The listing builds one solid part. Answer for the finished solid, in the listing's coordinates (mm). A direction names the side the tool comes from. Give positions to 0.01 mm unless a question says otherwise; leave off trailing zeros. Order: outer loops, then holes, each group sorted by start corner. A loop starts at its lowest first (then second) coordinate and runs counter-clockwise, first axis right, second up.
```python
from build123d import *

# Parameters (mm, degrees)
SKETCH1_W           = 57
SKETCH1_H           = 5
BOSS_EXTRUDE1_DEPTH = 30
SKETCH2_W           = 30
SKETCH2_H           = 8
BOSS_EXTRUDE2_DEPTH = 47
SKETCH3_R           = 5
CUT_EXTRUDE1_DEPTH  = 80.737067917
SKETCH5_R           = 1.6
CUT_EXTRUDE3_DEPTH  = 14
FILLET1_R           = 5
FILLET2_R           = 5


with BuildPart() as part:
    # Sketch1 → Boss-Extrude1 (new body)
    with BuildSketch(Plane(origin=(0, 0, 0), x_dir=(0, 0, -1), z_dir=(1, 0, 0))):
        with Locations((28.5, 2.5)):
            Rectangle(SKETCH1_W, SKETCH1_H)
    boss_extrude1 = extrude(amount=BOSS_EXTRUDE1_DEPTH)

    # Sketch2 → Boss-Extrude2 (add)
    with BuildSketch(Plane(origin=(0, 5, 0), x_dir=(1, 0, 0), z_dir=(0, 1, 0))):
        with Locations((15, 53)):
            Rectangle(SKETCH2_W, SKETCH2_H)
    extrude(amount=BOSS_EXTRUDE2_DEPTH)

    # Sketch3 → Cut-Extrude1 (cut, through all)
    with BuildSketch(Plane(origin=(0, 5, 0), x_dir=(1, 0, 0), z_dir=(0, 1, 0))):
        with Locations(Location((15, 22, 0), (0, 0, 270))):
            Circle(SKETCH3_R)
    cut_extrude1 = extrude(amount=-CUT_EXTRUDE1_DEPTH, mode=Mode.SUBTRACT)

    # Sketch5 → Cut-Extrude3 (cut)
    with BuildSketch(Plane(origin=(0, 52, 0), x_dir=(1, 0, 0), z_dir=(0, 1, 0))):
        with Locations(Location((5, 53, 0), (0, 0, 270))):
            Circle(SKETCH5_R)
        with Locations(Location((25, 53, 0), (0, 0, 270))):
            Circle(SKETCH5_R)
    extrude(amount=-CUT_EXTRUDE3_DEPTH, mode=Mode.SUBTRACT)

    # Fillet1
    fillet1_edges = [part.edges().sort_by_distance(p)[0] for p in [
        (15, 5, -49),
        (30, 2.5, 0),
        (0, 2.5, 0),
        (15, 0, -57),
    ]]
    fillet(fillet1_edges, radius=FILLET1_R)

    # Mirror1: Boss-Extrude1, Cut-Extrude1 across plane
    add(boss_extrude1.mirror(Plane(origin=(0, 0, -53), x_dir=(1, 0, 0), z_dir=(0, 0, -1))))
    add(cut_extrude1.mirror(Plane(origin=(0, 0, -53), x_dir=(1, 0, 0), z_dir=(0, 0, -1))), mode=Mode.SUBTRACT)

    # Fillet2
    fillet2_edges = [part.edges().sort_by_distance(p)[0] for p in [
        (15, 5, -57),
        (0, 2.5, -106),
        (30, 2.5, -106),
    ]]
    fillet(fillet2_edges, radius=FILLET2_R)


solid = part.part
```
1) Straight lines are drawn through the part: probe 1 along X at (y, z) = (49, -53); probe 2 along X at (y, z) = (2, -22); probe 3 along Z at (x, y) = (20, 44.5). For each, find the intervals that lie inside material, in ascending order.
Geometry says:
probe 1: x = 0 to 3.4, 6.6 to 23.4, 26.6 to 30
probe 2: x = 0 to 10, 20 to 30
probe 3: z = -57 to -49
2) Find section B-B (x = 15). Write down the section's boundary in (y, z), then the cut area to 3 significant figures.
Geometry says:
outline: (0, -106) - (5, -106) - (5, -89) - (0, -89) - close; (0, -79) - (5, -79) - (5, -62) arc R5 cw to (10, -57) - (52, -57) - (52, -49) - (10, -49) arc R5 cw to (5, -44) - (5, -27) - (0, -27) - close; (0, -17) - (5, -17) - (5, 0) - (0, 0) - close
area: 817 mm2
3) Find section A-A (z = -22). Write down the section's boundary in (x, y), then the cut area to 3 significant figures.
Geometry says:
outline: (0, 0) - (10, 0) - (10, 5) - (0, 5) - close; (20, 0) - (30, 0) - (30, 5) - (20, 5) - close
area: 100 mm2
4) For a pull along X with two mould halves and no side action, classify faces 1 (the cylindrical face through (1, 3, -2)), 2 (the cylindrical face through (15, 7, -48)), 3 (the flat face through (5, 38, -53)) as +X half, -X half, draft (parallel to the pull), parting line (faces both ways), or undercut.
Geometry says:
face 1: -X half
face 2: draft
face 3: undercut
5) Find section D-D (z = -53). Write down the section's boundary in (x, y).
Geometry says:
outline: (0, 0) - (30, 0) - (30, 52) - (26.6, 52) - (26.6, 38) - (23.4, 38) - (23.4, 52) - (6.6, 52) - (6.6, 38) - (3.4, 38) - (3.4, 52) - (0, 52) - close
6) Given P1, Ø15, axis at x = 12.5, z = -16.5, coming from the +Y side; P2, Ø3, axis at x = 3, y = 26.5, coming from the +Z side; P3, Ø6, axis at x = 12, y = 10, coming from the -Z side; P4, Ø10, axis at y = 14.5, z = -26.5, coming from the -X side (3 decimals), each flat-ended and moving along its own axis, determine where each tip first touches the part or whether it passes through.
Geometry says:
P1: stops at y = 5
P2: stops at z = -49
P3: stops at z = -58
P4: passes through
7) A tool of negligible diameter and unlimited length cuts with its end or side. For faces 4 (the flat face through (14.8, 5, -16.8)), 5 (the cylindrical face through (25.481, 45.098, -51.474)), 6 (the flat face through (15, 31, -57)), from which of +Z, -Z, +X, -X, +Y, -Y can it reach the whole face along a straight path? Write none if from no direction.
Geometry says:
face 4: +Z, +X, -X, +Y
face 5: +Y
face 6: -Z, +X, -X, +Y
8) Find section C-C (x = 21). Write down the section's boundary in (y, z), then the cut area to 3 significant figures.
Geometry says:
outline: (0, -106) - (5, -106) - (5, -62) arc R5 cw to (10, -57) - (52, -57) - (52, -49) - (10, -49) arc R5 cw to (5, -44) - (5, 0) - (0, 0) - close
area: 917 mm2
